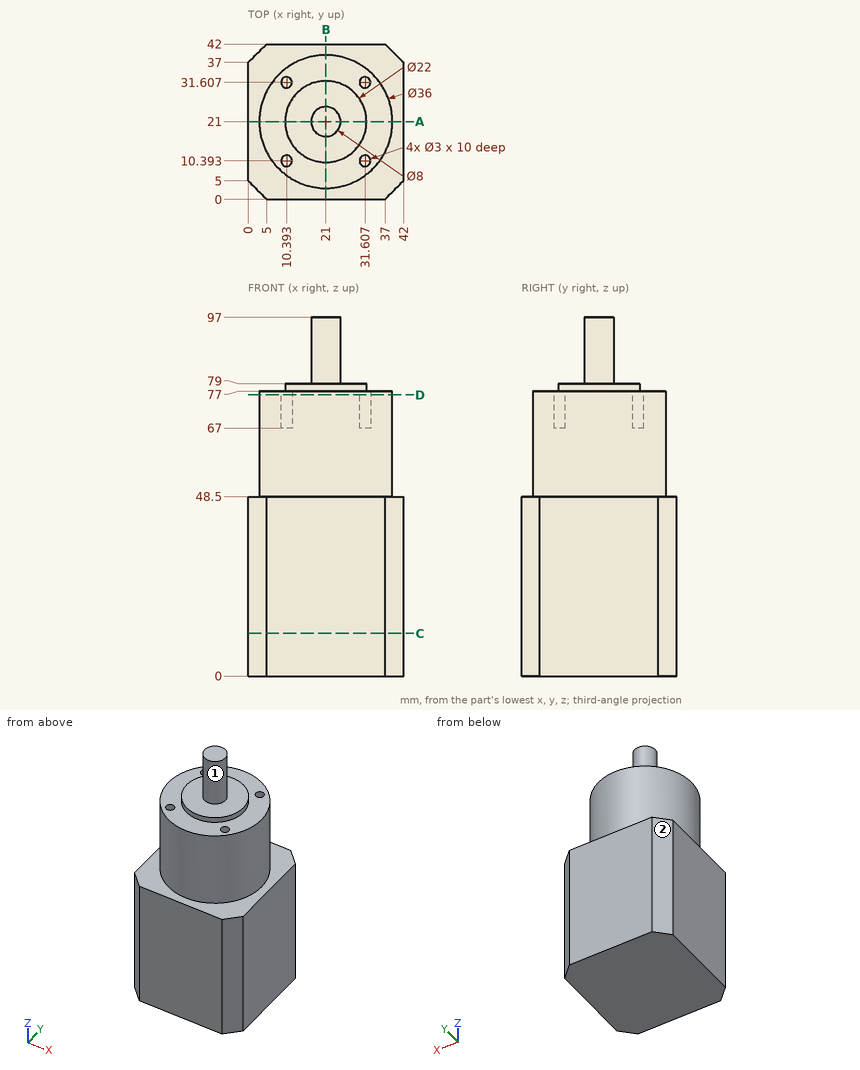
Verification items for this drawing (mm, ordinates from the low corner). A direction names the side the tool comes from. Coordinates: 2 decimals unless noted, no trailing zeros. Loops run counter-clockwise (first coordinate to the right, second up) from the corner with the lowest first, then second, coordinate; pieces in that order, holes last.
Item 1: Sectioned sample at C-C, the plane z = 11.5. Record the boundary of the cut face in (x, y), then the cut area to 3 significant figures.
Item 2: Sectioned sample at A-A, the plane y = 21. Record the boundary of the cut face in (x, z), then the cut area to 3 significant figures.
Item 3: Access from +Z, -Z, +X, -X, +Y, -Y to the whole of each face (thin tool, end or side, straight path). Record for the marked faces 1 and 2.
Item 4: Go/stop test with flat-tipped pins: pin 1 Ø1.5 at (x, y) = (32, 10) entering from +Z; pin 2 Ø3.5 at (x, y) = (10.39, 31.61) entering from +Z; pin 3 Ø5 at (x, y) = (14, 19) entering from +Z; pin 4 Ø12 at (x, z) = (32, 85.5) entering from -Y. Record where each tip stops, or that it passes through.
Item 5: Sectioned sample at D-D, the plane z = 76. Record the boundary of the cut face in (x, y).
Item 6: Thickness scan on line 1 (Z direction, x = 9, y = 3); line 2 (Z direction, x = 12, y = 16.5); line 3 (X direction, y = 40, z = 33). Record the ranges inside material, lowest first.
Check result:
1. outline: (0, 5) - (5, 0) - (37, 0) - (42, 5) - (42, 37) - (37, 42) - (5, 42) - (0, 37) - close
1. area: 1,710 mm2
2. outline: (0, 0) - (42, 0) - (42, 48.5) - (39, 48.5) - (39, 77) - (32, 77) - (32, 79) - (25, 79) - (25, 97) - (17, 97) - (17, 79) - (10, 79) - (10, 77) - (3, 77) - (3, 48.5) - (0, 48.5) - close
2. area: 3,250 mm2
3. face 1: +Z
3. face 2: +Z, -Z, -X, +Y
4. pin 1: stops at z = 67
4. pin 2: stops at z = 77
4. pin 3: stops at z = 79
4. pin 4: passes through
5. outline: circle Ø36 at (21, 21); hole circle Ø3 at (10.39, 10.39); hole circle Ø3 at (10.39, 31.61); hole circle Ø3 at (31.61, 10.39); hole circle Ø3 at (31.61, 31.61)
6. line 1: z = 0 to 48.5
6. line 2: z = 0 to 79
6. line 3: x = 3 to 39
